Can you work these out from the drawing? Everything is in mm from the part's minimum corner. A direction names the side the tool comes from. Round coordinates to 2 decimals unless told otherwise and drop trailing zeros. Loops run counter-clockwise (first coordinate to the right, second up) from the corner with the lowest first, then second, coordinate; pieces in that order, holes last. Notation, with made-up numbers: (68.25, 68) - (117.25, 68) arc R27 cw to (117.25, 99) - close; hole circle Ø7 at (-28, 27.5). An arc over 180 degrees is marked (long way). Return JSON: item names as keys, results as strings. Group by question number.
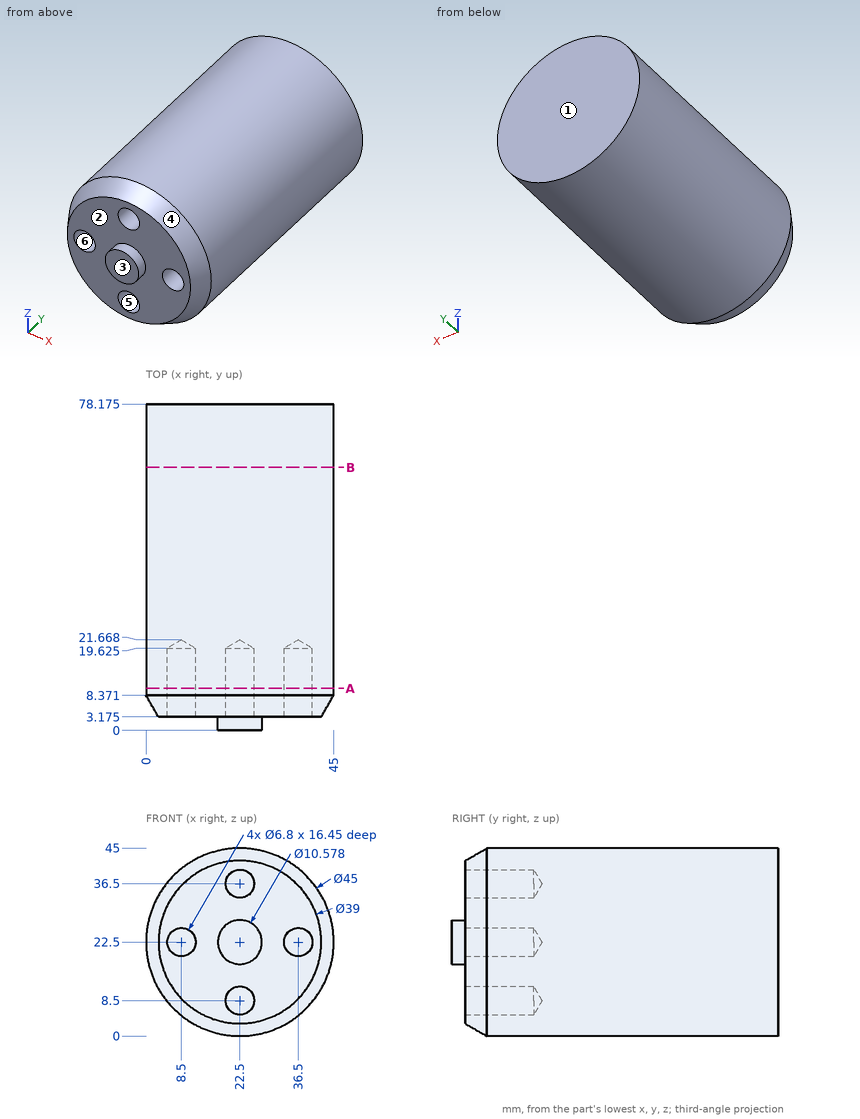
Q1. If we mould it in two halves opening along Z, with no side actions, what happens to the marked faces 3, 4, 5 and 6? For each: +Z half, -Z half, draft (parallel to the pull), parting line (faces both ways), or undercut.
Q2. Will these pins go through, and if not, where does the flat tip stop? pin 1 Ø19.5 at (x, z) = (29, 15) entering from -Y; pin 2 Ø12 at (x, y) = (24, 8.5) entering from -Z; pin 3 Ø2 at (x, y) = (39, 44.5) entering from -Z; pin 4 Ø1.5 at (y, z) = (13, 32.5) entering from +X.
Q3. For the marked faces 1 and 2, which set-ups out of +Z, -Z, +X, -X, +Y, -Y let a thin tool reach every point of the face, with its end or its side?
Q4. Imagine slicing it at B-B, the plane y = 63. List the corners of the cut face in (x, z) for me, and give its area (3 significant figures).
Q5. Please list where these lines run through material, in increasing order: line 1 (Z direction, x = 22.5, y = 13); line 2 (Z direction, x = 21.5, y = 13); line 3 (X direction, y = 6.5, z = 22) (1 decimal).
Q6. Imagine slicing it at A-A, the plane y = 10. List the corners of the cut face in (x, z) for me, and give its area (4 significant figures).
Output values:
{
 "1": {"face 3": "draft", "face 4": "parting line", "face 5": "undercut", "face 6": "undercut"},
 "2": {"pin 1": "stops at y = 0", "pin 2": "stops at z = 0", "pin 3": "stops at z = 6.19", "pin 4": "stops at x = 43.01"},
 "3": {"face 1": "+Z, -Z, +X, -X, +Y", "face 2": "-Y"},
 "4": {"outline": "circle Ø45 at (22.5, 22.5)", "area": "1,590 mm^2"},
 "5": {"line 1": "z = 0 to 5.1, 11.9 to 33.1, 39.9 to 45", "line 2": "z = 0.02 to 5.25, 11.75 to 33.25, 39.75 to 44.98", "line 3": "x = 1.1 to 5.1, 11.9 to 33.1, 39.9 to 43.9"},
 "6": {"outline": "circle Ø45 at (22.5, 22.5); hole circle Ø6.8 at (8.5, 22.5); hole circle Ø6.8 at (22.5, 8.5); hole circle Ø6.8 at (22.5, 36.5); hole circle Ø6.8 at (36.5, 22.5)", "area": "1,445 mm^2"}
}
